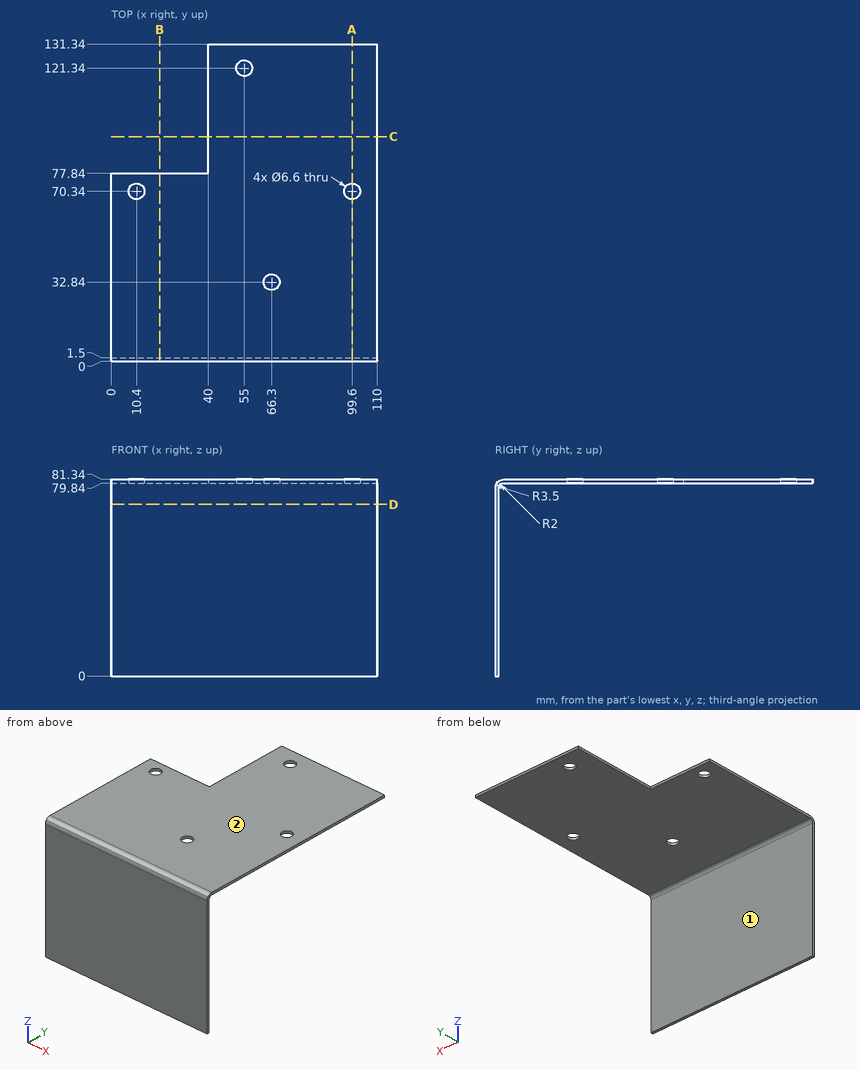
Print and shaded views of the part. All mm, measured from the part's lowest x, y and z. A direction names the side the tool comes from. Round coordinates to 2 decimals unless told otherwise and drop trailing zeros. Loops run counter-clockwise (first coordinate to the right, second up) from the corner with the lowest first, then second, coordinate; pieces in that order, holes last. Notation, with made-up numbers: M 22,42 L 32,42 A32 cw 32,74 Z; hole C 72.25,39 d10. An arc over 180 degrees is marked long. One line per question, with ' | ' between items.
1) Flat gauge pins, fed straight in: pin 1 (1.2 mm diameter, centred on y = 118, z = 80.5, fed in from -X); pin 2 (7.5 mm diameter, centred on x = 66.3, y = 32.84, fed in from -Z); pin 3 (5.5 mm diameter, centred on x = 99.6, y = 70.34, fed in from -Z); pin 4 (1.2 mm diameter, centred on x = 23, z = 81, fed in from +Y). Where does each tip first touch, or does it go through?
Solved:
pin 1: stops at x = 40 | pin 2: stops at z = 79.84 | pin 3: passes through | pin 4: stops at y = 77.84
2) Band-saw the part on D-D (z = 71). Give the cut face in (x, y), then the cut area to 3 significant figures.
Solved:
outline: M 0,0 L 110,0 L 110,1.5 L 0,1.5 Z | area: 165 mm²
3) 3-axis set-ups, long thin cutter, end or side, ignore diameter. For the marked faces 1 and 2: which of +Z, -Z, +X, -X, +Y, -Y reach the whole face in a straight line?
Solved:
face 1: -Z, +X, -X, +Y | face 2: +Z, +X, -X, +Y, -Y
4) Band-saw the part on B-B (x = 20). Give the cut face in (y, z), then the cut area to 3 significant figures.
Solved:
outline: M 0,0 L 1.5,0 L 1.5,77.84 A2 cw 3.5,79.84 L 77.84,79.84 L 77.84,81.34 L 3.5,81.34 A3.5 ccw 0,77.84 Z | area: 235 mm²
5) Band-saw the part on A-A (x = 99.6). Give the cut face in (y, z).
Solved:
outline: M 0,0 L 1.5,0 L 1.5,77.84 A2 cw 3.5,79.84 L 67.04,79.84 L 67.04,81.34 L 3.5,81.34 A3.5 ccw 0,77.84 Z; M 73.64,79.84 L 131.34,79.84 L 131.34,81.34 L 73.64,81.34 Z
6) Drill centre lines: line 1 along Z through (x, y) = (65.5, 107); line 2 along Y through (x, z) = (66.3, 80.35); line 3 along Y through (x, z) = (102, 30.5). Where is each one in solid material? Low to high.
Solved:
line 1: z = 79.84 to 81.34 | line 2: y = 1.06 to 29.54, 36.14 to 131.34 | line 3: y = 0 to 1.5
7) Band-saw the part on C-C (y = 93). Give the cut face in (x, z).
Solved:
outline: M 40,79.84 L 110,79.84 L 110,81.34 L 40,81.34 Z
